Read the model definition and answer for the solid it produces. Units are mm, in the model's axes. A direction names the side the tool comes from. Coordinates: 2 decimals unless noted, no trailing zeros. Loops run counter-clockwise (first coordinate to the right, second up) from the corner with the lowest first, then second, coordinate; pieces in that order, holes last. Notation, with made-up numbers: (-4.75, -11.75) -> (33.25, -11.75) arc R11 ccw to (33.25, 8.25) -> close; hole circle Ø2 at (87, -25.5). An arc over 180 degrees is marked (long way). Answer as CSV lines item,"result".
```python
from build123d import *

# Parameters (mm, degrees)
FILLET_R = 0.2


with BuildPart() as part:
    # Sketch → Revolution (revolve)
    with BuildSketch(Plane.XZ):
        Polygon((15, 75), (17, 71), (15, 71), (15, 41), (23.5, 41), (23.5, 0), (20.5, 0), (20.5, 26), (18.5, 26), (12.5, 39), (12.5, 75), align=None)
    revolve(axis=Axis((0, 0, 0), (0, 0, 1)))

    # Fillet
    fillet_edges = [part.edges().sort_by_distance(p)[0] for p in [
        (-17, 0, 71),
    ]]
    fillet(fillet_edges, radius=FILLET_R)


solid = part.part
```
Q1. A cutting plane is placed at D-D, the plane x = 19.5. Write down the section's boundary in (y, z), and give its area (3 significant figures).
Results:
outline,"(-13.11, 0) -> (-6.32, 0) -> (-6.32, 26) -> (6.32, 26) -> (6.32, 0) -> (13.11, 0) -> (13.11, 41) -> (-13.11, 41) -> close"
area,"747 mm²"
Q2. A cutting plane is placed at A-A, the plane x = 0. Write down the section's boundary in (y, z).
Results:
outline,"(-23.5, 0) -> (-20.5, 0) -> (-20.5, 26) -> (-18.5, 26) -> (-12.5, 39) -> (-12.5, 75) -> (-15, 75) -> (-16.86, 71.29) arc R0.2 ccw to (-16.68, 71) -> (-15, 71) -> (-15, 41) -> (-23.5, 41) -> close; (12.5, 39) -> (18.5, 26) -> (20.5, 26) -> (20.5, 0) -> (23.5, 0) -> (23.5, 41) -> (15, 41) -> (15, 71) -> (16.68, 71) arc R0.2 ccw to (16.86, 71.29) -> (15, 75) -> (12.5, 75) -> close"
Q3. A cutting plane is placed at C-C, the plane z = 62.5. Write down the section's boundary in (x, y), and give its area (3 significant figures).
Results:
outline,"circle Ø30 at (0, 0); hole circle Ø25 at (0, 0)"
area,"216 mm²"
Q4. Find the intervals of material crossed by probe 1 along Y at (x, z) = (0, 52.5); probe 2 along Y at (x, z) = (0, 20); probe 3 along Z at (x, y) = (-17, -15), in increasing order. Write a range as [from, to].
Results:
probe 1,"y = [-15, -12.5], [12.5, 15]"
probe 2,"y = [-23.5, -20.5], [20.5, 23.5]"
probe 3,"z = [0, 41]"
Q5. Given pin 1 Ø4 at (y, z) = (-18.5, 22.5) entering from -X; pin 2 Ø4 at (y, z) = (-12, 65.5) entering from +X; pin 3 Ø8 at (y, z) = (-18.5, 43.5) entering from +X; pin 4 Ø2 at (x, y) = (-13, -8) entering from +Z, each flat-ended and moving along its own axis, determine where each tip first touches the part or whether it passes through.
Results:
pin 1,"stops at x = -16.73"
pin 2,"stops at x = 11.18"
pin 3,"stops at x = 17.77"
pin 4,"stops at z = 75"
Q6. For a pull along X with two mould halves and no side action, classify faces 1 (the face through (11.923, 3.755, 57.252)), 2 (the face through (0.3, -15.3, 41)), 3 (the face through (-14.985, 0.66, 55.79)) as pulls with the +X half, pulls with the -X half, needs draft (parallel to the pull), parting line crosses it, or undercut.
Results:
face 1,"undercut"
face 2,"needs draft"
face 3,"parting line crosses it"
Q7. For faces 4 (the face through (-4.444, -20.013, 13.182)), 5 (the face through (-14, 6, 71)), 6 (the face through (2, 21, 0)), determine the directions among +Z, -Z, +X, -X, +Y, -Y from which every point of the face is accessible in a straight line to the end or side of a thin tool.
Results:
face 4,"-Z"
face 5,"none"
face 6,"-Z, +X, -X, +Y, -Y"
